```python
from build123d import *

# Parameters (mm, degrees)
F0_R     = 5
F1_DEPTH = 4
F2_R     = 5
F3_R     = 10


with BuildPart() as f1:
    # F0 (on Top) → F1 (new body)
    with BuildSketch(Plane.XY):
        Polygon((-60, 0), (0, 0), (0, 180), (-26.811556, 202.497566), (-62.164874, 160.365122), (-30, 133.375588), (-30, 30), (-60, 30), align=None)
        with Locations((-45, 15)):
            Circle(F0_R, mode=Mode.SUBTRACT)
        with Locations((-15, 15)):
            Circle(F0_R, mode=Mode.SUBTRACT)
        with Locations((-44.862615, 165.427913)):
            Circle(F0_R, mode=Mode.SUBTRACT)
        with Locations((-35.220801, 176.918579)):
            Circle(F0_R, mode=Mode.SUBTRACT)
        with Locations((-29.541727, 152.57216)):
            Circle(F0_R, mode=Mode.SUBTRACT)
        with Locations((-19.899912, 164.062827)):
            Circle(F0_R, mode=Mode.SUBTRACT)
        with Locations((-25.578987, 188.409246)):
            Circle(F0_R, mode=Mode.SUBTRACT)
        with Locations((-10.258098, 175.553494)):
            Circle(F0_R, mode=Mode.SUBTRACT)
    extrude(amount=F1_DEPTH)

    # F2
    f2_edges = [f1.edges().sort_by_distance(p)[0] for p in [
        (-62.164874, 160.365122, 2),
        (-26.811556, 202.497566, 2),
        (0, 180, 2),
        (0, 0, 2),
        (-60, 0, 2),
        (-60, 30, 2),
    ]]
    fillet(f2_edges, radius=F2_R)

    # F3
    f3_edges = [f1.edges().sort_by_distance(p)[0] for p in [
        (-30, 30, 2),
        (-30, 133.375588, 2),
    ]]
    fillet(f3_edges, radius=F3_R)


solid = f1.part
```
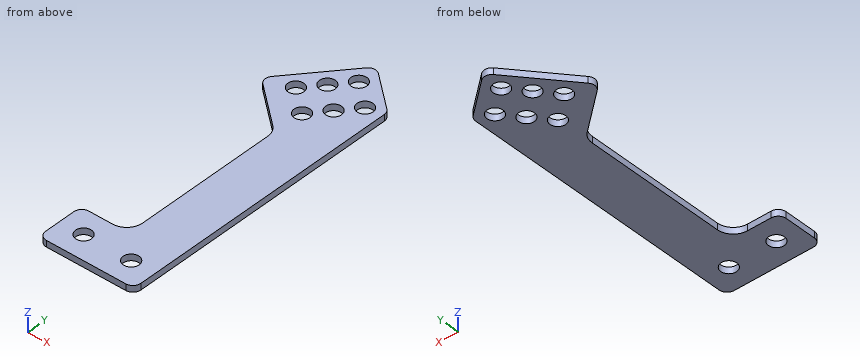
Input: part model. Units: mm. Frame: model coordinates. Give positions to 0.01 mm unless a question says otherwise; leave off trailing zeros. Order: outer loops, then holes, each group sorted by start corner. A loop starts at its lowest first (then second) coordinate and runs counter-clockwise, first axis right, second up.
1. Cut plane D-D (y = 114). Return loops of the section in (x, z).
Computed:
outline: (-30, 0) - (0, 0) - (0, 4) - (-30, 4) - close
2. Cut plane A-A (y = 15). Return loops of the section in (x, z).
Computed:
outline: (-60, 0) - (-50, 0) - (-50, 4) - (-60, 4) - close; (-40, 0) - (-20, 0) - (-20, 4) - (-40, 4) - close; (-10, 0) - (0, 0) - (0, 4) - (-10, 4) - close
3. Pin query (flat end, axial travel): pin 1 Ø8 at (x, y) = (-29.54, 152.57) entering from +Z; pin 2 Ø11.5 at (x, y) = (-44.86, 165.43) entering from +Z; pin 3 Ø1.2 at (x, z) = (-49.5, 1.5) entering from +Y; pin 4 Ø1.5 at (y, z) = (67.5, 1.5) entering from -X. Return the tip coordinate at first contact, or that it passes through.
Computed:
pin 1: passes through
pin 2: stops at z = 4
pin 3: stops at y = 176.17
pin 4: stops at x = -30
4. Line query: probe 1 along Y at (x, z) = (-45, 1.25); probe 2 along Y at (x, z) = (-10.5, 0.35); probe 3 along Y at (x, z) = (-43, 2.2). Output: solid intervals per line, ascending.
Computed:
probe 1: y = 0 to 10, 20 to 30, 145.96 to 160.43, 170.43 to 180.82
probe 2: y = 0 to 12.82, 17.18 to 170.56, 180.55 to 188.81
probe 3: y = 0 to 10.42, 19.58 to 30, 144.28 to 160.79, 170.07 to 183.2
5. Cut plane B-B (x = -45). Return loops of the section in (y, z).
Computed:
outline: (0, 0) - (10, 0) - (10, 4) - (0, 4) - close; (20, 0) - (30, 0) - (30, 4) - (20, 4) - close; (145.96, 0) - (160.43, 0) - (160.43, 4) - (145.96, 4) - close; (170.43, 0) - (180.82, 0) - (180.82, 4) - (170.43, 4) - close
6. Cut plane C-C (z = 1.45). State how many separate pieces and enclosed holes the cut face has, and give its area (3 significant figures).
Computed:
separate pieces: 1
enclosed holes: 8
area: 7,090 mm2
